```python
from build123d import *

# Parameters (mm, degrees)
ESQUISSE1_R             = 4
BOSS_EXTRU_1_DEPTH      = 3
ENL_V_MAT_EXTRU_1_REACH = 51.7
ESQUISSE2_W             = 5.860148805
ESQUISSE2_H             = 10.034501378
ESQUISSE2_H_2           = 10.034501379


with BuildPart() as part:
    # Esquisse1 → Boss.-Extru.1 (new body)
    with BuildSketch(Plane.XY):
        with BuildLine():
            Line((-11.661538462, 23.484615385), (-11.661538462, -3.515384615))
            Line((-11.661538462, -3.515384615), (-1.661538462, -3.515384615))
            Line((-1.661538462, -3.515384615), (-1.661538462, -6.515384615))
            Line((-1.661538462, -6.515384615), (-11.661538462, -6.515384615))
            Line((-11.661538462, -6.515384615), (-11.661538462, -11.515384615))
            Line((-11.661538462, -11.515384615), (2.059303641, -11.515384615))
            Line((2.059303641, -11.515384615), (32.110271991, 0.723219922))
            ThreePointArc((32.110271991, 0.723219922), (38.338461538, 9.984615385), (32.110271991, 19.246010847))
            Line((32.110271991, 19.246010847), (2.059303641, 31.484615385))
            Line((2.059303641, 31.484615385), (-11.661538462, 31.484615385))
            Line((-11.661538462, 31.484615385), (-11.661538462, 26.484615385))
            Line((-11.661538462, 26.484615385), (-1.661538462, 26.484615385))
            Line((-1.661538462, 26.484615385), (-1.661538462, 23.484615385))
            Line((-1.661538462, 23.484615385), (-11.661538462, 23.484615385))
        make_face()
        with Locations((28.338461538, 9.984615385)):
            Circle(ESQUISSE1_R, mode=Mode.SUBTRACT)
    extrude(amount=BOSS_EXTRU_1_DEPTH)

    # Esquisse2 → Enlèv. mat.-Extru.1 (cut, up to next)
    with BuildSketch(Plane.XY.offset(3), mode=Mode.PRIVATE) as enl_v_mat_extru_1_sk1:
        with Locations((-9.591612865, 30.1046068)):
            Rectangle(ESQUISSE2_W, ESQUISSE2_H)
    enl_v_mat_extru_1_tool1 = extrude(enl_v_mat_extru_1_sk1.sketch, amount=-ENL_V_MAT_EXTRU_1_REACH, mode=Mode.PRIVATE) & part.part
    # Esquisse2 → Enlèv. mat.-Extru.1 (cut, up to next)
    with BuildSketch(Plane.XY.offset(3), mode=Mode.PRIVATE) as enl_v_mat_extru_1_sk2:
        with Locations((-9.591612865, -10.135376031)):
            Rectangle(ESQUISSE2_W, ESQUISSE2_H_2)
    enl_v_mat_extru_1_tool2 = extrude(enl_v_mat_extru_1_sk2.sketch, amount=-ENL_V_MAT_EXTRU_1_REACH, mode=Mode.PRIVATE) & part.part
    add(enl_v_mat_extru_1_tool1.solids().sort_by_distance((-9.591613, 30.104607, 3))[0], mode=Mode.SUBTRACT)
    add(enl_v_mat_extru_1_tool2.solids().sort_by_distance((-9.591613, -10.135376, 3))[0], mode=Mode.SUBTRACT)


solid = part.part
```
Here's how the part is built. I have some questions about the finished solid (model axes, mm). A direction names the side the tool comes from. Coordinates: 2 decimals unless noted, no trailing zeros. Order: outer loops, then holes, each group sorted by start corner. A loop starts at its lowest first (then second) coordinate and runs counter-clockwise, first axis right, second up.
1) Imagine slicing it at D-D on y = 0. List the corners of the cut face in (x, z) for me.
2) We'd pull the mould along X, two halves only. Please class faces 4 (the face through (-6.662, -9, 2)), 5 (the face through (16.874, -5.482, 1.479)), 6 (the face through (24.342, 10.16, 1.479)), 7 (the face through (-7, 23.485, 1)): +X half, -X half, draft (parallel to the pull), parting line (faces both ways), or undercut.
3) Will these pins go through, and if not, where does the flat tip stop? pin 1 (0.9 mm diameter, centred on y = -8.5, z = 1.5, fed in from -X); pin 2 (1 mm diameter, centred on x = 25.5, z = 2.5, fed in from -Y).
4) I need wall thicknesses on line 1 (Y direction, x = -6, z = 0.5); line 2 (Y direction, x = 28.5, z = 2.3); line 3 (X direction, y = 12.5, z = 0.4). Which ranges of each line are inside material? Lowest first, please.
5) Imagine slicing it at A-A on x = 26. List the corners of the cut face in (y, z) for me.
6) Which directions (+Z, -Z, +X, -X, +Y, -Y) give clear straight access to the entire face, cutting with the end or side of a thin tool? Please do faces 1 (the face through (-6.662, 29, 2)), 2 (the face through (-1.662, -5, 1)), 3 (the face through (13, 10, 0)).
7) Imagine slicing it at B-B on z = 1.35. List the corners of the cut face in (x, y) for me.
8) Imagine slicing it at C-C on y = 11.5. List the corners of the cut face in (x, z) for me, and give its area (3 significant figures).
Response values:
1. outline: (-11.66, 0) - (30.33, 0) - (30.33, 3) - (-11.66, 3) - close
2. face 4: -X half
2. face 5: +X half
2. face 6: undercut
2. face 7: draft
3. pin 1: stops at x = -6.66
3. pin 2: stops at y = -2.17
4. line 1: y = -11.52 to -6.52, -3.52 to 23.48, 26.48 to 31.48
4. line 2: y = -0.75 to 5.99, 13.98 to 20.72
4. line 3: x = -11.66 to 25.23, 31.45 to 38.02
5. outline: (-1.77, 0) - (6.74, 0) - (6.74, 3) - (-1.77, 3) - close; (13.23, 0) - (21.73, 0) - (21.73, 3) - (13.23, 3) - close
6. face 1: +Z, -Z, -X, +Y
6. face 2: +Z, -Z, -X
6. face 3: -Z, +X, -X, +Y, -Y
7. outline: (-11.66, -3.52) - (-1.66, -3.52) - (-1.66, -6.52) - (-6.66, -6.52) - (-6.66, -11.52) - (2.06, -11.52) - (32.11, 0.72) arc R10 ccw to (32.11, 19.25) - (2.06, 31.48) - (-6.66, 31.48) - (-6.66, 26.48) - (-1.66, 26.48) - (-1.66, 23.48) - (-11.66, 23.48) - close; hole circle Ø8 at (28.34, 9.98)
8. outline: (-11.66, 0) - (24.64, 0) - (24.64, 3) - (-11.66, 3) - close; (32.04, 0) - (38.22, 0) - (38.22, 3) - (32.04, 3) - close
8. area: 127 mm2
